Geometry check sheet. Reference: drawing and pictorial views, mm from the part's lowest x, y, z. A direction names the side the tool comes from. Round coordinates to 2 decimals unless told otherwise and drop trailing zeros. Loops run counter-clockwise (first coordinate to the right, second up) from the corner with the lowest first, then second, coordinate; pieces in that order, holes last. Notation, with made-up numbers: (82, 44) - (126, 44) arc R34 ccw to (126, 79) - close; hole circle Ø7 at (67.5, 68.5). An arc over 180 degrees is marked (long way). Answer as CSV lines item,"result". Start each with the question number.
1) Thickness scan on line 1 along Y through (x, z) = (4.55, 4.8) (3 decimals); line 2 along Y through (x, z) = (3, 22.5); line 3 along Z through (x, y) = (7.25, 24.5). Record the ranges inside material, lowest first.
2) Cross-section at B-B on z = 20. Record the boundary of the cut face in (x, y), and give its area (3 significant figures).
3) Depth check by flat-ended pin: P1, Ø1, axis at x = 8, z = 27, coming from the -Y side; P2, Ø2.5, axis at y = 16.775, z = 4.8, coming from the -X side; P3, Ø1.7, axis at x = 8, z = 20.5, coming from the +Y side; P4, Ø2.5, axis at x = 9, y = 16, coming from the -Z side. Enter the tip coordinate at first touch or a pass-through.
4) Access from +Z, -Z, +X, -X, +Y, -Y to the whole of each face (thin tool, end or side, straight path). Record for the marked faces 1, 2 and 3.
5) Cross-section at C-C on y = 25.5. Record the boundary of the cut face in (x, z).
6) Cross-section at D-D on x = 9. Record the boundary of the cut face in (y, z).
7) Cross-section at A-A on z = 4.8. Record the boundary of the cut face in (x, y) (3 decimals).
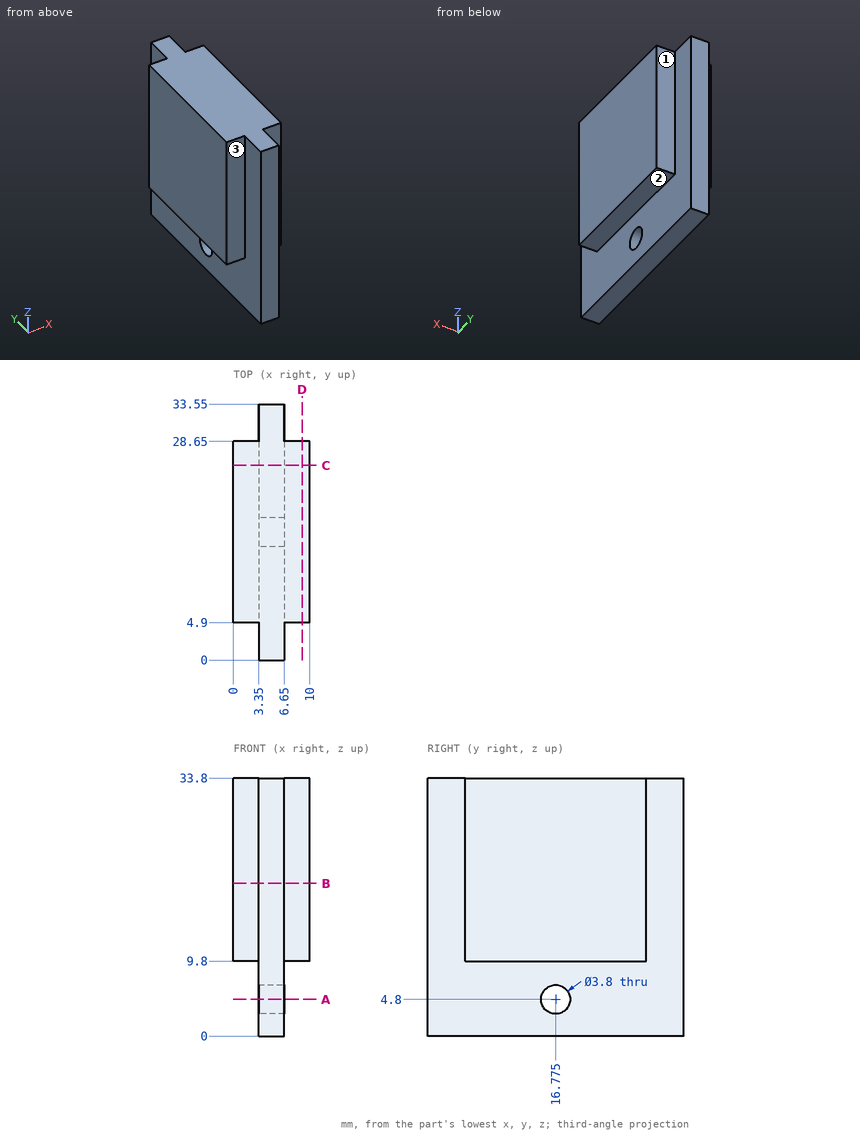
Answer block:
1,line 1,"y = 0 to 14.875, 18.675 to 33.55"
1,line 2,"y = 4.9 to 28.65"
1,line 3,"z = 9.8 to 33.8"
2,outline,"(0, 4.9) - (3.35, 4.9) - (3.35, 0) - (6.65, 0) - (6.65, 4.9) - (10, 4.9) - (10, 28.65) - (6.65, 28.65) - (6.65, 33.55) - (3.35, 33.55) - (3.35, 28.65) - (0, 28.65) - close"
2,area,"270 mm^2"
3,P1,"stops at y = 4.9"
3,P2,"passes through"
3,P3,"stops at y = 28.65"
3,P4,"stops at z = 9.8"
4,face 1,"+Z, -Z, +X, +Y"
4,face 2,"-Z, +X, +Y, -Y"
4,face 3,"+Z, -Z, -X, -Y"
5,outline,"(0, 9.8) - (3.35, 9.8) - (3.35, 0) - (6.65, 0) - (6.65, 9.8) - (10, 9.8) - (10, 33.8) - (0, 33.8) - close"
6,outline,"(4.9, 9.8) - (28.65, 9.8) - (28.65, 33.8) - (4.9, 33.8) - close"
7,outline,"(3.35, 0) - (6.65, 0) - (6.65, 14.875) - (3.35, 14.875) - close; (3.35, 18.675) - (6.65, 18.675) - (6.65, 33.55) - (3.35, 33.55) - close"
